```python
from build123d import *

# Parameters (mm, degrees)
F0_R     = 5.5
F0_R_2   = 2.25
F1_DEPTH = 13.5
F2_R     = 5.5
F2_R_2   = 3
F3_DEPTH = 12.5
F4_R     = 3
F4_R_2   = 2.75
F5_DEPTH = 6


with BuildPart() as f1:
    # F0 (on Top) → F1 (new body)
    with BuildSketch(Plane.XY):
        Circle(F0_R)
        Circle(F0_R_2, mode=Mode.SUBTRACT)
    extrude(amount=F1_DEPTH)

    # F2 (on face) → F3 (cut)
    with BuildSketch(Plane.XY.offset(13.5)):
        Circle(F2_R)
        Circle(F2_R_2, mode=Mode.SUBTRACT)
    extrude(amount=-F3_DEPTH, mode=Mode.SUBTRACT)

    # F4 (on face) → F5 (cut)
    with BuildSketch(Plane.XY.offset(13.5)):
        Circle(F4_R)
        Circle(F4_R_2, mode=Mode.SUBTRACT)
    extrude(amount=-F5_DEPTH, mode=Mode.SUBTRACT)


solid = f1.part
```
CAD build for the part. Positions are in the model's coordinates, mm. A direction names the side the tool comes from. Round coordinates to 2 decimals unless told otherwise and drop trailing zeros. Order: outer loops, then holes, each group sorted by start corner. A loop starts at its lowest first (then second) coordinate and runs counter-clockwise, first axis right, second up. Notation, with made-up numbers: (40.5, 77.25) - (76.5, 77.25) arc R15 ccw to (76.5, 95.25) - close; hole circle Ø2 at (15, 39.5). An arc over 180 degrees is marked (long way). Answer as CSV lines item,"result". Start each with the question number.
1. Saw through at C-C, the plane z = 10.5. Write the cut outline in (x, y).
2. Saw through at D-D, the plane y = -4.5. Write the cut outline in (x, z).
3. Tool access for faces 1 (the face through (-0.596, -2.685, 10.542)), 2 (the face through (-0.29, 2.23, 6.66)): list every direction of +Z, -Z, +X, -X, +Y, -Y with a clear straight run to the whole face (end or side of a thin tool).
4. Saw through at A-A, the plane y = 0. Write the cut outline in (x, z), and give its area (4 significant figures).
5. Drill centre lines: L1, parallel to Y at x = 0, z = 8; L2, parallel to Z at x = -3, y = 3; L3, parallel to Y at x = -0.75, z = 12.5. Where is each one in solid material? Low to high. Write a range as [from, to].
6. Pin check, flat tips, straight feed: pin 1 (3 mm diameter, centred on x = 0, z = 11.5, fed in from -Y); pin 2 (6 mm diameter, centred on x = -1, z = 8.5, fed in from +Y); pin 3 (1 mm diameter, centred on y = 4, z = 6.5, fed in from +X). Stop position of each tip, or through.
Model answer:
1,outline,"circle Ø5.5 at (0, 0); hole circle Ø4.5 at (0, 0)"
2,outline,"(-3.16, 0) - (3.16, 0) - (3.16, 1) - (-3.16, 1) - close"
3,face 1,"+Z"
3,face 2,"+Z, -Z"
4,outline,"(-5.5, 0) - (-2.25, 0) - (-2.25, 13.5) - (-2.75, 13.5) - (-2.75, 7.5) - (-3, 7.5) - (-3, 1) - (-5.5, 1) - close; (2.25, 0) - (5.5, 0) - (5.5, 1) - (3, 1) - (3, 7.5) - (2.75, 7.5) - (2.75, 13.5) - (2.25, 13.5) - close"
4,area,"22.25 mm²"
5,L1,"y = [-2.75, -2.25], [2.25, 2.75]"
5,L2,"z = [0, 1]"
5,L3,"y = [-2.65, -2.12], [2.12, 2.65]"
6,pin 1,"stops at y = -2.75"
6,pin 2,"stops at y = 3"
6,pin 3,"passes through"
